Autodesk Inventor part; units mm, degrees
ref_plane "YZ Plane" through (0, 0, 0) normal (1, 0, 0) x (0, 1, 0)
ref_plane "XZ Plane" through (0, 0, 0) normal (0, 1, 0) x (-1, 0, 0)
ref_plane "XY Plane" through (0, 0, 0) normal (0, 0, 1) x (1, 0, 0)
sketch "Skizze1" plane through (0, 0, 0) normal (0, 0, 1) x (1, 0, 0)
  line L0 (-11.2, 0) -> (11.2, 0)
  line L1 (0, -11.2) -> (0, 11.2)
  circle A0 centre (0, 0) radius 8
  dimension "d0" = 16
extrude "Extrusion1" add sketch "Skizze1" along normal blind 19.5
sketch "Skizze2" plane through (0, 0, 0) normal (0, 1, 0) x (-1, 0, 0)
  line L0 (11.2, 0) -> (-11.2, 0)
  line L1 (0, -3.9) -> (0, 23.4)
  arc A0 (-3.5, -5) -> (3.5, -5) centre (0, -5) ccw
  line L2 (3.5, -5) -> (3.5, 0)
  line L3 (-8, 0) -> (8, 0)
  line L4 (-3.5, -5) -> (-3.5, 0)
  point P0 (0, 0)
  dimension "d3" = 3.5
  dimension "d4" = 5
extrude "Extrusion2" add sketch "Skizze2" along normal mid plane 3
sketch "Skizze3" plane through (0, 1.5, 0) normal (0, 1, 0) x (1, 0, 0)
  arc A0 (3.5, 5) -> (-3.5, 5) centre (0, 5) ccw
  point P0 (0, 0)
hole "Bohrung1" at (0, 1.5, -5) direction (0, -1, 0) diameter 3 end through all
sketch "Skizze4" plane through (0, 0, 0) normal (0, 0, -1) x (-1, 0, 0)
  line L0 (-3.5, -1.5) -> (-3.5, 1.5)
  line L1 (3.5, -1.5) -> (3.5, 1.5)
  line L2 (-3.5, 1.5) -> (3.5, 1.5)
  line L3 (-3.5, -1.5) -> (-3.5, 1.5)
  line L4 (3.5, -1.5) -> (-3.5, -1.5)
  arc A0 (-3.1623, 1.5) -> (-3.1623, -1.5) centre (0, 0) ccw
  line L5 (-3.1623, 1.5) -> (-3.8633, 1.5)
  line L6 (-3.8633, 1.5) -> (-3.8633, -1.5)
  line L7 (-3.8633, -1.5) -> (-3.1623, -1.5)
  dimension "d14" = 3.5
  dimension "d15" = 3.8632
sketch "Skizze5" plane through (0, -1.5, 0) normal (0, -1, 0) x (1, 0, 0)
  arc A0 (-3.5, -5) -> (3.5, -5) centre (0, -5) ccw
  arc A1 (-3.5, -5) -> (3.5, -5) centre (0, -5) ccw
  line L0 (-3.5, 0) -> (-3.5, -5)
  line L1 (3.5, -5) -> (3.5, 0.5133)
  point P0 (0, 0)
sketch3d "3D-Skizze1"
  line L0 (3.5, -1.5, 0) -> (3.5, -1.5, -5)
  arc A0 (-3.5, -1.5, -5) -> (-2.4749, -1.5, -7.4749) centre (0, -1.5, -5) ccw
  arc A1 (-2.4749, -1.5, -7.4749) -> (0, -1.5, -8.5) centre (0, -1.5, -5) ccw
  arc A2 (0, -1.5, -8.5) -> (2.4749, -1.5, -7.4749) centre (0, -1.5, -5) ccw
  arc A3 (2.4749, -1.5, -7.4749) -> (3.5, -1.5, -5) centre (0, -1.5, -5) ccw
  line L1 (-3.5, -1.5, -5) -> (-3.5, -1.5, 0)
sweep "Sweeping1" cut profiles "Skizze4" path "3D-Skizze1" contours L7 L6 L5 L0 | L0 A0 L4 | L0 L2 A0
properties part number "Kolben"
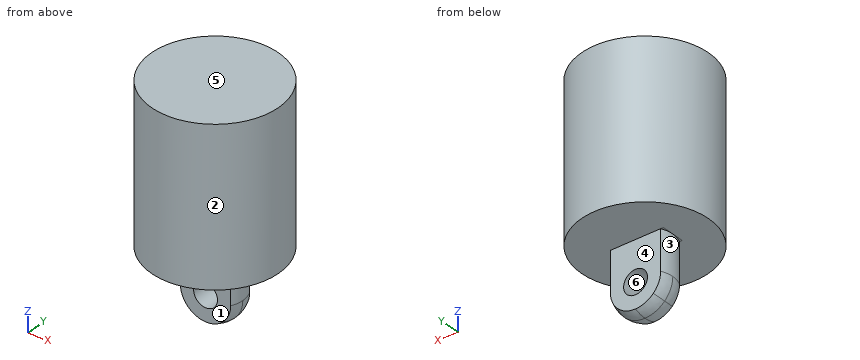
CAD build for the part. Positions are in the model's coordinates, mm. Face numbers are marked on the shaded views. A direction names the side the tool comes from. Round coordinates to 2 decimals unless told otherwise and drop trailing zeros. Loops run counter-clockwise (first coordinate to the right, second up) from the corner with the lowest first, then second, coordinate; pieces in that order, holes last. Notation, with made-up numbers: M -22,28 L -1,28 A35 ccw -1,62 Z; hole C 78.5,30.5 d8. An arc over 180 degrees is marked long. Use a Markdown table: item, result. Add a question column.
(1) Which spindle directions (+Z, -Z, +X, -X, +Y, -Y) get a long thin tool onto all of the face, cutting with end or side? Do the marked faces 1, 2 and 3. Say none if no direction does.
(2) Cut at C-C (x = 4.75). Give the cut face in (y, z), and give its area (3 significant figures).
(3) Cut at A-A (z = 11.5). Give the cut face in (x, y), and give its area (3 significant figures).
(4) Cut at B-B (y = -2). Give the cut face in (x, z), and give its area (3 significant figures).
(5) Pull direction Z, two halves, no side cores. Call the marked faces 4, 5 and 6: +Z half, -Z half, draft (parallel to the pull), parting line (faces both ways), or undercut.
(6) Flat gauge pins, fed straight in: pin 1 (4 mm diameter, centred on y = -3.5, z = 0, fed in from +X); pin 2 (3 mm diameter, centred on x = -4.5, z = 14, fed in from -Y); pin 3 (1.5 mm diameter, centred on x = 1.5, z = 12.5, fed in from +Y). Where does each tip first touch, or does it go through?
(7) Drill centre lines: line 1 (X direction, y = 0, z = -5); line 2 (Z direction, x = 4.5, y = 6.25); line 3 (X direction, y = 0.7, z = -5). Where is each one in solid material? Low to high.
Geometry says:
| question | item | result |
|---|---|---|
| 1 | face 1 | -Z, +X, -X, -Y |
| 1 | face 2 | +Z, -Z |
| 1 | face 3 | -Z, -X |
| 2 | outline | M -6.44,0 L 6.44,0 L 6.44,19.5 L -6.44,19.5 Z |
| 2 | area | 251 mm² |
| 3 | outline | C 0,0 d16 |
| 3 | area | 201 mm² |
| 4 | outline | M -7.75,0 L 7.75,0 L 7.75,19.5 L -7.75,19.5 Z |
| 4 | area | 302 mm² |
| 5 | face 4 | draft |
| 5 | face 5 | +Z half |
| 5 | face 6 | undercut |
| 6 | pin 1 | stops at x = 7.86 |
| 6 | pin 2 | stops at y = -7.42 |
| 6 | pin 3 | stops at y = 7.96 |
| 7 | line 1 | x = -3.5 to -1.5, 1.5 to 3.5 |
| 7 | line 2 | z = 0 to 19.5 |
| 7 | line 3 | x = -3.43 to -1.5, 1.5 to 3.43 |
